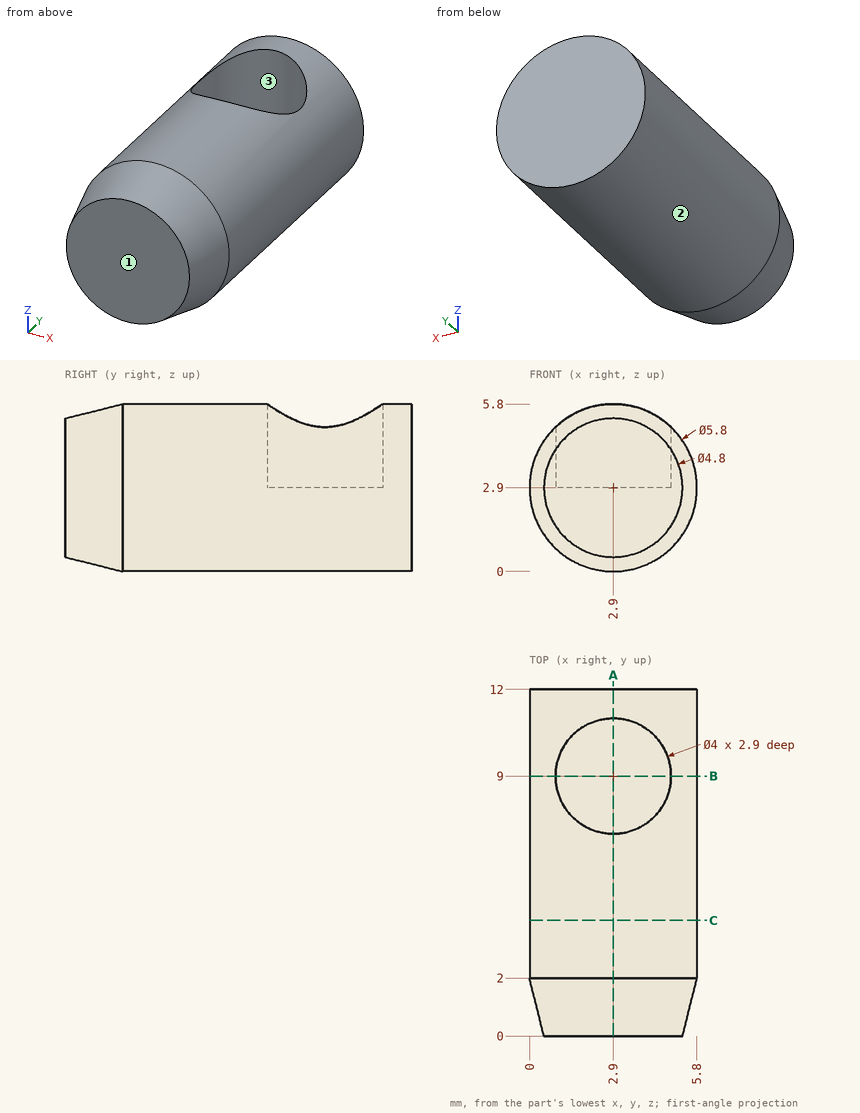
Verification items for this drawing (mm, ordinates from the low corner). Coordinates: 2 decimals unless noted, no trailing zeros. Write each loop counter-clockwise with the first axis right and the second up, starting at its lowest first coordinate (ties: lowest second). Pieces come first, ordered by that corner, then holes. Notation, with made-up numbers: M 0.25,-32.5 L 33.25,-32.5 A27 ccw 33.25,-4.5 Z; hole C 68,-4.5 d2. An arc over 180 degrees is marked long. Use CSV: the item, a comma, the result in double quotes.
Q1. Section check B-B, the plane y = 9. Enter the section's corners in (x, z), and give its area (3 significant figures).
Computed values:
outline,"M 0.9,2.9 L 0.9,5 A2.9 ccw long 4.9,5 L 4.9,2.9 Z"
area,"15.8 mm²"
Q2. Section check A-A, the plane x = 2.9. Enter the section's corners in (y, z), and give its area (3 significant figures).
Computed values:
outline,"M 0,0.5 L 2,0 L 12,0 L 12,5.8 L 11,5.8 L 11,2.9 L 7,2.9 L 7,5.8 L 2,5.8 L 0,5.3 Z"
area,"57.0 mm²"
Q3. Mould release check, pull along X, two halves, no side actions. Record for the marked faces 1, 2 and 3: pulls with the +X half, pulls with the -X half, needs draft (parallel to the pull), parting line crosses it, or undercut.
Computed values:
face 1,"needs draft"
face 2,"parting line crosses it"
face 3,"undercut"
Q4. Go/stop test with flat-tipped pins: P1, Ø3, axis at x = 2.5, y = 10, coming from the +Z side; P2, Ø1.5, axis at x = 2, y = 10, coming from the -Z side. Record where each tip stops, or that it passes through.
Computed values:
P1,"z = 5.8"
P2,"z = 0"
Q5. Thickness scan on line 1 along Y through (x, z) = (2.9, 4.15); line 2 along X through (y, z) = (9, 4.2); line 3 along X through (y, z) = (8.25, 4.9). Record the ranges inside material, lowest first. Write a range as [from, to].
Computed values:
line 1,"[0, 7], [11, 12]"
line 2,"[0.31, 0.9], [4.9, 5.49]"
line 3,"[0.8, 1.05], [4.75, 5]"
Q6. Section check C-C, the plane y = 4. Enter the section's corners in (x, z), and give its area (3 significant figures).
Computed values:
outline,"C 2.9,2.9 d5.8"
area,"26.4 mm²"
